The listing builds one solid part. Answer for the finished solid, in the listing's coordinates (mm). Face numbers are marked on the shaded views. A direction names the side the tool comes from. Give positions to 0.01 mm unless a question says otherwise; leave off trailing zeros. Order: outer loops, then holes, each group sorted by start corner. A loop starts at its lowest first (then second) coordinate and runs counter-clockwise, first axis right, second up. Notation, with made-up numbers: (46, -17.5) - (75, -17.5) arc R11 cw to (75, -6.5) - close; hole circle Ø4 at (-15, 70.25). An arc over 180 degrees is marked (long way). Use CSV: the item, a comma, the result in double quotes.
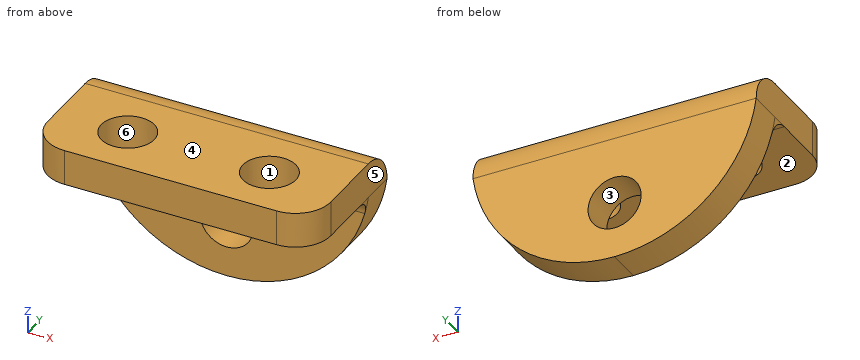
```python
from build123d import *

# Parameters (mm, degrees)
BOSS_EXTRUDE4_DEPTH = 16
CUT_EXTRUDE3_DEPTH  = 16
SKETCH16_R          = 1.5
CUT_EXTRUDE4_DEPTH  = 16
FILLET1_R           = 2
FILLET2_R           = 2
SKETCH17_R          = 1.5
CUT_EXTRUDE5_DEPTH  = 16
FILLET3_R           = 1


with BuildPart() as part:
    # Sketch14 → Boss-Extrude4 (new body)
    with BuildSketch(Plane(origin=(0, 0, 0), x_dir=(0, 0, -1), z_dir=(1, 0, 0))):
        Polygon((11.48032087, -6.121921179), (9.48032087, -6.121921179), (9.48032087, 1.878078821), (18.48032087, 1.878078821), (18.48032087, -0.121921179), (11.48032087, -0.121921179), align=None)
    extrude(amount=BOSS_EXTRUDE4_DEPTH)

    # Sketch15 → Cut-Extrude3 (cut)
    with BuildSketch(Plane.XZ.offset(0.121921179)):
        with BuildLine():
            ThreePointArc((8, -18.48032087), (2.684927094, -16.483261335), (0, -11.48032087))
            Line((0, -11.48032087), (0, -18.48032087))
            Line((0, -18.48032087), (8, -18.48032087))
        make_face()
        with BuildLine():
            Line((16, -18.48032087), (16, -11.48032087))
            ThreePointArc((16, -11.48032087), (13.315072906, -16.483261335), (8, -18.48032087))
            Line((8, -18.48032087), (16, -18.48032087))
        make_face()
    extrude(amount=-CUT_EXTRUDE3_DEPTH, mode=Mode.SUBTRACT)

    # Sketch16 → Cut-Extrude4 (cut)
    with BuildSketch(Plane.XY.offset(-9.48032087)):
        with Locations((4, -3.121921179)):
            Circle(SKETCH16_R)
        with Locations((12, -3.121921179)):
            Circle(SKETCH16_R)
    extrude(amount=-CUT_EXTRUDE4_DEPTH, mode=Mode.SUBTRACT)

    # Fillet1
    fillet1_edges = [part.edges().sort_by_distance(p)[0] for p in [
        (16, -6.121921179, -10.48032087),
        (0, -6.121921179, -10.48032087),
    ]]
    fillet(fillet1_edges, radius=FILLET1_R)

    # Fillet2
    fillet2_edges = [part.edges().sort_by_distance(p)[0] for p in [
        (8, 1.878078821, -9.48032087),
    ]]
    fillet(fillet2_edges, radius=FILLET2_R)

    # Sketch17 → Cut-Extrude5 (cut)
    with BuildSketch(Plane(origin=(0, 1.878078821, 0), x_dir=(1, 0, 0), z_dir=(0, 1, 0))):
        with Locations(Location((8, 15.28032087, 0), (0, 0, 270))):
            Circle(SKETCH17_R)
    extrude(amount=-CUT_EXTRUDE5_DEPTH, mode=Mode.SUBTRACT)

    # Fillet3
    # the kernel refuses this fillet: 1 mm, written as the material it adds along each edge
    with BuildSketch(Plane(origin=(0, -0.121921179, -11.48032087), x_dir=(0, -1, 0), z_dir=(1, 0, 0))) as fillet3_piece_1_section:
        with BuildLine():
            CenterArc((FILLET3_R, FILLET3_R), FILLET3_R, 180, 90)
            Line((0, FILLET3_R), (0, 0))
            Line((0, 0), (FILLET3_R, 0))
        make_face()
    fillet3_piece_1 = extrude(amount=16, mode=Mode.PRIVATE)
    fillet3_piece_1 = fillet3_piece_1 & Plane(origin=(8, -0.348905362, -10.408892299), x_dir=(0, 0, -1), z_dir=(0, -1, 0)) * Cylinder(8.071428571, 36, mode=Mode.PRIVATE)
    add(fillet3_piece_1)


solid = part.part
```
Item 1: The part is cut by section C-C (y = -2.25). Give the vertices of the cut face in (x, z), and give its area (3 significant figures).
Taken from the geometry:
outline,"(0, -11.48) - (2.78, -11.48) - (2.78, -9.48) - (0, -9.48) - close; (5.22, -11.48) - (10.78, -11.48) - (10.78, -9.48) - (5.22, -9.48) - close; (13.22, -11.48) - (16, -11.48) - (16, -9.48) - (13.22, -9.48) - close"
area,"22.2 mm^2"
Item 2: Find the intervals of material crossed by line 1 along X through (y, z) = (-2.75, -10); line 2 along Y through (x, z) = (10.75, -16.75); line 3 along X through (y, z) = (0, -14.75), in increasing order.
Taken from the geometry:
line 1,"0 to 2.55, 5.45 to 10.55, 13.45 to 16"
line 2,"-0.12 to 1.88"
line 3,"1.2 to 6.6, 9.4 to 14.8"
Item 3: The part is cut by section B-B (x = 12.25). Give the vertices of the cut face in (y, z).
Taken from the geometry:
outline,"(-6.12, -11.48) - (-4.6, -11.48) - (-4.6, -9.48) - (-6.12, -9.48) - close; (-1.64, -11.48) - (-1.12, -11.48) arc R1 cw to (-0.12, -12.48) - (-0.12, -17.27) - (1.88, -17.27) - (1.88, -11.48) arc R2 ccw to (-0.12, -9.48) - (-1.64, -9.48) - close"
Item 4: The part is cut by section D-D (z = -16). Give the vertices of the cut face in (x, y).
Taken from the geometry:
outline,"(2.18, -0.12) - (6.68, -0.12) - (6.68, 1.88) - (2.18, 1.88) - close; (9.32, -0.12) - (13.82, -0.12) - (13.82, 1.88) - (9.32, 1.88) - close"
Item 5: The mould has two halves that part along X. Classify the marked faces 3, 4, 5 and 6: +X half, -X half, draft (parallel to the pull), parting line (faces both ways), or undercut.
Taken from the geometry:
face 3,"undercut"
face 4,"draft"
face 5,"+X half"
face 6,"undercut"
Item 6: The part is cut by section A-A (z = -14.25). Give the vertices of the cut face in (x, y).
Taken from the geometry:
outline,"(0.9, -0.12) - (6.91, -0.12) - (6.91, 1.88) - (0.9, 1.88) - close; (9.09, -0.12) - (15.1, -0.12) - (15.1, 1.88) - (9.09, 1.88) - close"
Item 7: Each of these flat-tipped pins is pushed along its axis until it touches: pin 1 (4 mm diameter, centred on x = 9, y = -3.5, fed in from -Z); pin 2 (5 mm diameter, centred on x = 10.5, z = -16, fed in from -Y). Where does it stop, or does it pass through?
Taken from the geometry:
pin 1,"z = -11.48"
pin 2,"y = -0.12"
Item 8: Which of the six approach directions +Z, -Z, +X, -X, +Y, -Y give full straight-line access (tool end or side, diameter ignored) to the marked faces 1 and 2?
Taken from the geometry:
face 1,"+Z, -Z"
face 2,"-Z, +X, -X, -Y"
